Verification items for the finished model (mm, model axes). A direction names the side the tool comes from. Round coordinates to 2 decimals unless told otherwise and drop trailing zeros. Write each loop counter-clockwise with the first axis right and the second up, starting at its lowest first coordinate (ties: lowest second). Pieces come first, ordered by that corner, then holes.
from build123d import *

# Parameters (mm, degrees)
SKETCH1_R               = 1.25
BOSS_EXTRUDE1_DEPTH     = 2
BOSS_EXTRUDE2_DEPTH     = 7.5
SKETCH3_R               = 1.25
CUT_EXTRUDE1_DEPTH      = 2
CUT_EXTRUDE1_DEPTH_BACK = 4
SKETCH4_W               = 5
SKETCH4_H               = 2
SKETCH4_W_2             = 4.2
SKETCH4_H_2             = 1.2
CUT_EXTRUDE2_DEPTH      = 4


with BuildPart() as part:
    # Sketch1 → Boss-Extrude1 (new body)
    with BuildSketch(Plane.XY):
        Polygon((1952.176808721, 1466.884115951), (1957.176808721, 1466.884115951), (1957.176808721, 1462.884115951), (1958.426808721, 1462.884115951), (1958.426808721, 1458.884115951), (1957.176808721, 1458.884115951), (1957.176808721, 1454.884115951), (1952.176808721, 1454.884115951), (1952.176808721, 1458.884115951), (1950.926808721, 1458.884115951), (1950.926808721, 1462.884115951), (1952.176808721, 1462.884115951), align=None)
        with Locations((1954.676808721, 1460.884115951)):
            Circle(SKETCH1_R, mode=Mode.SUBTRACT)
    extrude(amount=BOSS_EXTRUDE1_DEPTH)

    # Sketch2 → Boss-Extrude2 (add)
    with BuildSketch(Plane.ZY.offset(-1950.926808721)):
        with BuildLine():
            Line((2, 1458.884115951), (2, 1459.884115951))
            ThreePointArc((2, 1459.884115951), (2.292893219, 1459.17700917), (3, 1458.884115951))
            Line((3, 1458.884115951), (2, 1458.884115951))
        make_face()
        with BuildLine():
            Line((0, 1458.884115951), (-1, 1458.884115951))
            ThreePointArc((-1, 1458.884115951), (-0.292893219, 1459.17700917), (0, 1459.884115951))
            Line((0, 1459.884115951), (0, 1458.884115951))
        make_face()
    extrude(amount=-BOSS_EXTRUDE2_DEPTH)

    # Sketch3 → Cut-Extrude1 (cut, two sides)
    with BuildSketch(Plane.XY.offset(2)) as cut_extrude1_sk:
        with Locations((1954.676808721, 1460.884115951)):
            Circle(SKETCH3_R)
    extrude(amount=CUT_EXTRUDE1_DEPTH, mode=Mode.SUBTRACT)
    extrude(cut_extrude1_sk.sketch, amount=-CUT_EXTRUDE1_DEPTH_BACK, mode=Mode.SUBTRACT)

    # Sketch4 → Cut-Extrude2 (cut)
    with BuildSketch(Plane(origin=(0, 1466.884115951, 0), x_dir=(1, 0, 0), z_dir=(0, 1, 0))):
        with Locations((1954.676808721, -1)):
            Rectangle(SKETCH4_W, SKETCH4_H)
        with Locations((1954.676808721, -1)):
            Rectangle(SKETCH4_W_2, SKETCH4_H_2, mode=Mode.SUBTRACT)
    extrude(amount=-CUT_EXTRUDE2_DEPTH, mode=Mode.SUBTRACT)


solid = part.part
Q1. Tool access check on faces 4 (the flat face through (1955, 1457, 2)), 5 (the flat face through (1956.777, 1465, 1)), 6 (the flat face through (1954.7, 1462.4, 2)). Record the directions out of +Z, -Z, +X, -X, +Y, -Y that give a thin tool (end or side, any length) a straight path to the whole face; none if there is none.
Recorded:
face 4: +Z, +X, -X, -Y
face 5: +Z, -Z, +X, +Y
face 6: +Z, +X, -X, +Y
Q2. Sectioned sample at B-B (x = 1951.75). Enter the section's corners in (y, z).
Recorded:
outline: (1458.88, -1) arc R1 cw to (1459.88, 0) - (1462.88, 0) - (1462.88, 2) - (1459.88, 2) arc R1 cw to (1458.88, 3) - close
Q3. Depth check by flat-ended pin: P1, Ø1.5, axis at x = 1956.5, y = 1461.5, coming from the -Z side; P2, Ø1.2, axis at x = 1955, y = 1464.5, coming from the -Z side; P3, Ø3, axis at x = 1954.5, y = 1456.5, coming from the +Z side. Enter the tip coordinate at first touch or a pass-through.
Recorded:
P1: stops at z = 0
P2: stops at z = 0.4
P3: stops at z = 2
Q4. Material ranges on line 1 along Y through (x, z) = (1957, 1.75); line 2 along Z through (x, y) = (1953, 1462.75); line 3 along X through (y, z) = (1458.5, 1.45), recorded low to high.
Recorded:
line 1: y = 1454.88 to 1462.88
line 2: z = 0 to 2
line 3: x = 1952.18 to 1957.18
Q5. Sectioned sample at D-D (x = 1953). Enter the section's corners in (y, z), plus the area to 3 significant figures.
Recorded:
outline: (1454.88, 0) - (1458.88, 0) - (1458.88, -1) arc R1 cw to (1459.88, 0) - (1462.88, 0) - (1462.88, 0.4) - (1466.88, 0.4) - (1466.88, 1.6) - (1462.88, 1.6) - (1462.88, 2) - (1459.88, 2) arc R1 cw to (1458.88, 3) - (1458.88, 2) - (1454.88, 2) - close
area: 21.2 mm2
Q6. Sectioned sample at A-A (z = 1.25). Enter the section's corners in (x, y).
Recorded:
outline: (1950.93, 1458.88) - (1952.18, 1458.88) - (1952.18, 1454.88) - (1957.18, 1454.88) - (1957.18, 1458.88) - (1958.43, 1458.88) - (1958.43, 1462.88) - (1956.78, 1462.88) - (1956.78, 1466.88) - (1952.58, 1466.88) - (1952.58, 1462.88) - (1950.93, 1462.88) - close; hole circle Ø2.5 at (1954.68, 1460.88)
Q7. Release check for a two-part mould opening along Y. For faces 1 (the flat face through (1955, 1454.884, 1)), 2 (the flat face through (1958.427, 1461, 1)), 3 (the cylindrical face through (1953.685, 1460.124, 0.986)) record: released by +Y, released by -Y, zero draft, split by the parting line, or undercut.
Recorded:
face 1: released by -Y
face 2: zero draft
face 3: undercut
Q8. Sectioned sample at C-C (y = 1465.25). Enter the section's corners in (x, z).
Recorded:
outline: (1952.58, 0.4) - (1956.78, 0.4) - (1956.78, 1.6) - (1952.58, 1.6) - close
